The listing builds one solid part. Answer for the finished solid, in the listing's coordinates (mm). Face numbers are marked on the shaded views. A direction names the side the tool comes from. Round coordinates to 2 decimals unless told otherwise and drop trailing zeros. Write each loop counter-clockwise with the first axis right and the second up, starting at its lowest first coordinate (ties: lowest second). Pieces come first, ordered by that corner, then holes.
from build123d import *

# Parameters (mm, degrees)
SKETCH_1_R          = 8
EXTRUDE_1_DEPTH     = 29
CUT_EXTRUDE_1_DEPTH = 21


with BuildPart() as part:
    # 草图1 → 凸台-拉伸1 (new, symmetric)
    with BuildSketch(Plane.XY):
        with BuildLine():
            Line((35, 60), (17.367283762, -4.730856402))
            ThreePointArc((17.367283762, -4.730856402), (0, -18.000098543), (-17.367283762, -4.730856402))
            Line((-17.367283762, -4.730856402), (-35, 60))
            Line((-35, 60), (-35, 80))
            Line((-35, 80), (35, 80))
            Line((35, 80), (35, 60))
        make_face()
        with Locations(Location((0, 0, 0), (0, 0, 180))):
            Circle(SKETCH_1_R, mode=Mode.SUBTRACT)
    extrude(amount=EXTRUDE_1_DEPTH, both=True)

    # 草图2 → 切除-拉伸1 (cut, symmetric)
    with BuildSketch(Plane.XY):
        with BuildLine():
            Line((-35, 60), (35, 60))
            Line((35, 60), (17.367283762, -4.730856402))
            ThreePointArc((17.367283762, -4.730856402), (0, -18.000098543), (-17.367283762, -4.730856402))
            Line((-17.367283762, -4.730856402), (-35, 60))
        make_face()
    extrude(amount=CUT_EXTRUDE_1_DEPTH, both=True, mode=Mode.SUBTRACT)


solid = part.part
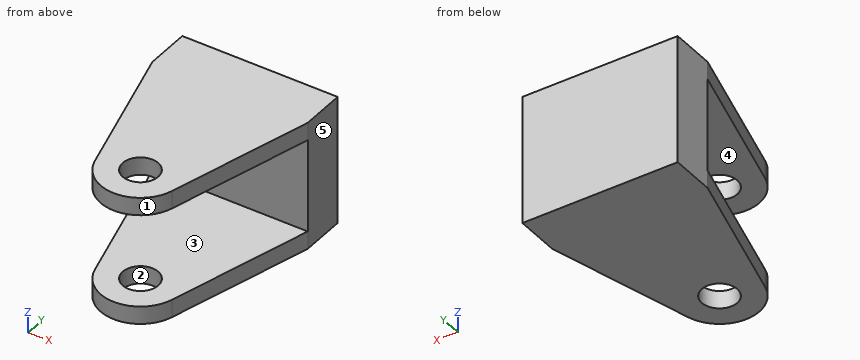
1. Given pin 1 (3 mm diameter, centred on x = 27.5, z = 16, fed in from -Y); pin 2 (8 mm diameter, centred on y = -7.5, z = -22.5, fed in from +X); pin 3 (4 mm diameter, centred on x = 14.5, z = -21, fed in from -Y), each flat-ended and moving along its own axis, determine where each tip first touches the part or whether it passes through.
Geometry says:
pin 1: stops at y = 60
pin 2: stops at x = 17.7
pin 3: stops at y = -12.95
2. A tool of negligible diameter and unlimited length cuts with its end or side. For the marked faces 4 and 5, from which of +Z, -Z, +X, -X, +Y, -Y can it reach the whole face along a straight path? Write none if from no direction.
Geometry says:
face 4: +X, -X, -Y
face 5: +Z, -Z, +X, +Y, -Y
3. For a pull along Y with two mould halves and no side action, classify the marked faces 1, 2 and 3 as released by +Y, released by -Y, zero draft, split by the parting line, or undercut.
Geometry says:
face 1: released by -Y
face 2: undercut
face 3: zero draft
4. Section D-D on y = 1.5 is taken. Determine the outline of the cut face in (x, z).
Geometry says:
outline: (-19.06, -29) - (-7.86, -29) - (-7.86, -21) - (-19.06, -21) - close; (-19.06, 21) - (-7.86, 21) - (-7.86, 29) - (-19.06, 29) - close; (7.86, -29) - (19.06, -29) - (19.06, -21) - (7.86, -21) - close; (7.86, 21) - (19.06, 21) - (19.06, 29) - (7.86, 29) - close
5. Section A-A on x = 0 is taken. Determine the outline of the cut face in (y, z).
Geometry says:
outline: (-18, -29) - (-8, -29) - (-8, -21) - (-18, -21) - close; (-18, 21) - (-8, 21) - (-8, 29) - (-18, 29) - close; (8, -29) - (80, -29) - (80, 29) - (8, 29) - (8, 21) - (60, 21) - (60, -21) - (8, -21) - close
6. Straight lines are drawn through the part: line 1 along Y through (x, z) = (0, -23); line 2 along Z through (x, y) = (-8, 40); line 3 along Y through (x, z) = (22, -2.5). For each, find the intervals that lie inside material, in ascending order.
Geometry says:
line 1: y = -18 to -8, 8 to 80
line 2: z = -29 to -21, 21 to 29
line 3: y = 60 to 80
7. Section C-C on y = 53.5 is taken. Determine the outline of the cut face in (x, z), plus the area to 3 significant figures.
Geometry says:
outline: (-33.23, -29) - (33.23, -29) - (33.23, -21) - (-33.23, -21) - close; (-33.23, 21) - (33.23, 21) - (33.23, 29) - (-33.23, 29) - close
area: 1,060 mm2
8. Section B-B on z = 23 is taken. Determine the outline of the cut face in (x, y), plus the area to 3 significant figures.
Geometry says:
outline: (-35, 60) - (-17.37, -4.73) arc R18 ccw to (17.37, -4.73) - (35, 60) - (35, 80) - (-35, 80) - close; hole circle Ø16 at (0, 0)
area: 4,930 mm2
